The listing builds one solid part. Answer for the finished solid, in the listing's coordinates (mm). A direction names the side the tool comes from. Coordinates: 2 decimals unless noted, no trailing zeros. Loops run counter-clockwise (first coordinate to the right, second up) from the corner with the lowest first, then second, coordinate; pieces in that order, holes last. Notation, with made-up numbers: M 68,-32.75 L 123,-32.75 A13 cw 123,-18.75 Z; hole C 78,-17 d7. An arc over 180 degrees is marked long. Answer as a JSON object with one key per item and string values. Group by question number.
1. Determine the mould class of faces 1 (the face through (6.1, -1.1, 0.9)), 2 (the face through (12.7, 0, 0)), 3 (the face through (-2.154, -0.605, -1.029)) for opening direction Y: released by +Y, released by -Y, zero draft, split by the parting line, or undercut.
2. For faces 4 (the face through (-2, 1.194, 0)), 5 (the face through (0, 2, 0)), 6 (the face through (-2.845, -1, 1)), determine the directions among +Z, -Z, +X, -X, +Y, -Y from which every point of the face is accessible in a straight line to the end or side of a thin tool.
3. A cutting plane is placed at A-A on x = 1. Give the vertices of the cut face in (y, z), and give its area (3 significant figures).
4. Given pin 1 (1 mm diameter, centred on x = 7.5, z = -1.5, fed in from -Y); pin 2 (1.5 mm diameter, centred on x = 10.5, y = 0, fed in from -Z); pin 3 (0.7 mm diameter, centred on x = -2.5, z = -0.5, fed in from -Y), each flat-ended and moving along its own axis, determine where each tip first touches the part or whether it passes through.
5. Straight lines are drawn through the part: L1, parallel to X at y = 0.25, z = 1.8; L2, parallel to Z at x = -1.5, y = -0.1; L3, parallel to Y at x = -1.75, z = -0.75. For each, find the intervals that lie inside material, in ascending order.
Autodesk Inventor part; units mm, degrees
ref_plane "Work Plane1" through (29, 0, 0) normal (0, -1, 0) x (1, 0, 0)
ref_plane "YZ Plane" through (0, 0, 0) normal (1, 0, 0) x (0, 1, 0)
ref_plane "XZ Plane" through (0, 0, 0) normal (0, 1, 0) x (-1, 0, 0)
sketch "Sketch1" plane through (0, 0, 0) normal (0, 0, 1) x (1, 0, 0)
  line L0 (-0.7535, 0) -> (12.7, 0)
  line L1 (12.7, 0) -> (12.7, 1.4224)
  line L2 (12.7, 1.4224) -> (1.5877, 1.4224)
  line L3 (1.5877, 1.4224) -> (0.0001, 1.4224)
  line L4 (0.0001, 1.4224) -> (0, 1.4224)
  line L5 (0, 1.4224) -> (0, 2.3241)
  line L6 (0, 2.3241) -> (-2.8448, 2.3241)
  line L7 (-2.8448, 2.3241) -> (-2.8448, 1.3785)
  line L8 (-2.8448, 1.3785) -> (-1.5494, 1.3785)
  line L9 (-1.5494, 1.3785) -> (-0.7535, 0)
  line L10 (-5.9538, 0) -> (15.809, 0)
  line L11 (0, -0.4648) -> (0, 2.7889)
  line L12 (1.5877, 1.4224) -> (0, 1.4224) construction
  dimension "d1" = 11.1123
  dimension "d2" = 1.5876
  dimension "d3" = 2.8448
  dimension "d4" = 1.2954
  dimension "d5" = 60
  dimension "d6" = 2.8448
  dimension "d7" = 2.8448
  dimension "d8" = 2.757
  dimension "d9" = 4.6482
  dimension "d26" = 12.7
revolve "Body" add sketch "Sketch1" angle 360 about axis through (-0.7535, 0, 0) along (1, 0, 0)
sketch "Sketch2" plane through (-2.8448, 0, 0) normal (-1, 0, 0) x (0, 0, 1)
  circle A0 centre (0, 0) radius 1.3785
  line L0 (0, -3.2537) -> (0, 3.2537)
  line L1 (-3.2537, 0) -> (3.2537, 0)
  line L2 (1.3785, 0) -> (0.6892, -1.1938)
  line L3 (0.6892, -1.1938) -> (-0.6892, -1.1938)
  line L4 (-0.6892, -1.1938) -> (-1.3785, 0)
  line L5 (-1.3785, 0) -> (-0.6892, 1.1938)
  line L6 (-0.6892, 1.1938) -> (0.6892, 1.1938)
  line L7 (0.6892, 1.1938) -> (1.3785, 0)
  point P0 (0, 0)
extrude "Slot" add sketch "Sketch2" against normal up to next contours L7 A0 | A0 L2 | L6 L0 A0 | A0 L0 L3 | L0 L6 A0 | A0 L3 L0 | L4 A0 | A0 L5
fillet "Fillet1" radius 0.2286 1 edges at (-2.8448, -2.3241, 0)
thread "Thread"
chamfer "Chamfer1" distance 0.3785 distance2 0.3785 1 edges at (12.7, -1.4224, 0) measured on face at (12.7, -0.2537, -0.5191)
ref_plane "Work Plane1" through (29, 0, 0) normal (0, -1, 0) x (1, 0, 0)
fillet "Fillet2" radius 0.1016 1 edges at (0.0001, -1.4224, 0)
equation "\"d1\" = GEL"
equation "\"d3\" = KOH"
equation "\"d4\" = INTI"
equation "\"d6\" = GD"
equation "\"d7\" = BDM"
equation "\"d8\" = 1.1547 * SW"
equation "\"d9\" = KOD"
equation "\"d26\" = NLG"
equation "\"d30\" = R"
equation "\"d17\" = RR"
equation "\"d13\" = GEL"
equation "\"d15\" = -0.5 * SPD + 0.5 * GD"
equation "\"d16\" = GUL"
equation "\"GD\" = 2.8448"
equation "\"NLG\" = 12.7"
equation "\"GEL\" = 11.1123"
equation "\"KOD\" = 4.6482"
equation "\"KOH\" = 2.8448"
equation "\"INTI\" = 1.2954"
equation "\"GAL\" = 1.5875"
equation "\"GUL\" = 0.37846"
equation "\"BDM\" = 2.8448"
equation "\"SW\" = 2.3876"
equation "\"RR\" = 0.2286"
equation "\"SPD\" = 2.08788"
equation "\"R\" = 0.1016"
equation "\"PHH\" = 0.127"
equation "\"GD1\" = SPD"
equation "\"THREADDIA\" = 2.8448"
equation "\"FAWI\" = 45deg"
equation "\"KOH1\" = 2.5654"
equation "\"NND\" = 2.8448"
equation "\"TOA\" = 30deg"
equation "\"E0\" = 1.155 * SW"
properties part number "ANSI B18.3 - No. 4 - 40 UNC - 1/2 HS HCS" material "Steel, Mild"
From the geometry:
{
 "1": {"face 1": "split by the parting line", "face 2": "zero draft", "face 3": "undercut"},
 "2": {"face 4": "-X", "face 5": "+X", "face 6": "+Z, -Z, -X, +Y, -Y"},
 "3": {"outline": "C 0,0 d2.84", "area": "6.36 mm²"},
 "4": {"pin 1": "stops at y = -1.01", "pin 2": "stops at z = -1.42", "pin 3": "stops at y = -2.32"},
 "5": {"L1": "x = -2.84 to 0", "L2": "z = -2.32 to -1.29, 1.29 to 2.32", "L3": "y = -2.2 to -1.09, 1.09 to 2.2"}
}
